Could you check a few things on this model? Use its own coordinates, in mm. A direction names the side the tool comes from. Coordinates: 2 decimals unless noted, no trailing zeros. Write each loop counter-clockwise with the first axis right and the second up, starting at its lowest first coordinate (ties: lowest second). Pieces come first, ordered by that corner, then holes.
```python
from build123d import *

# Parameters (mm, degrees)
SKETCH3_W          = 10
SKETCH3_H          = 1.5
CHAMFER1_SIZE      = 0.45
CUT_EXTRUDE1_DEPTH = 1.19


with BuildPart() as part:
    # Sketch3 → Revolve1 (revolve)
    with BuildSketch(Plane(origin=(0, 0, 0), x_dir=(0, 0, -1), z_dir=(1, 0, 0))):
        with Locations((0, 0.75)):
            Rectangle(SKETCH3_W, SKETCH3_H)
    revolve(axis=Axis((0, 0, -5), (0, 0, 1)))

    # Chamfer1
    chamfer1_edges = [part.edges().sort_by_distance(p)[0] for p in [
        (0, -1.5, -5),
    ]]
    chamfer(chamfer1_edges, length=CHAMFER1_SIZE)

    # Sketch6 → Revolve2 (revolve)
    with BuildSketch(Plane(origin=(0, 0, 0), x_dir=(0, 0, -1), z_dir=(1, 0, 0))):
        Polygon((-5, 3), (-4.8, 3), (-3.3, 1.5), (-3.3, 0), (-5, 0), align=None)
    revolve(axis=Axis((0, 0, -5), (0, 0, 1)))

    # Sketch8 → Cut-Extrude1 (cut)
    with BuildSketch(Plane.XY.offset(5)):
        Polygon((0, 1.154700538), (-1, 0.577350269), (-1, -0.577350269), (0, -1.154700538), (1, -0.577350269), (1, 0.577350269), align=None)
    extrude(amount=-CUT_EXTRUDE1_DEPTH, mode=Mode.SUBTRACT)

    # Cut-Extrude2 cone 1 section (through the dimple's axis) → Cut-Extrude2 (revolve, cut)
    with BuildSketch(Plane(origin=(0, 0, 5), x_dir=(0, -1, 0), z_dir=(1, 0, 0))):
        Polygon((0, 0), (1.154700538, 0), (0, 1.154700538), align=None)
    revolve(axis=Axis((0, 0, 5), (0, 0, -1)), mode=Mode.SUBTRACT)


solid = part.part
```
1. If we mould it in two halves opening along Y, with no side actions, what happens to faces 3 (the face through (0, 0, -5)), 4 (the face through (-0.07, -1.5, -0.68)), 5 (the face through (1, 0, 4))? For each: pulls with the +Y half, pulls with the -Y half, needs draft (parallel to the pull), parting line crosses it, or undercut.
Verdict:
face 3: needs draft
face 4: parting line crosses it
face 5: undercut
2. I want a section at A-A on y = 0. Please give me the cut outline in (x, z), plus the area to 3 significant figures.
Verdict:
outline: (-3, 4.8) - (-1.5, 3.3) - (-1.5, -4.55) - (-1.05, -5) - (1.05, -5) - (1.5, -4.55) - (1.5, 3.3) - (3, 4.8) - (3, 5) - (1.15, 5) - (1, 4.85) - (1, 3.81) - (-1, 3.81) - (-1, 4.85) - (-1.15, 5) - (-3, 5) - close
area: 30.2 mm2
3. On a 3-axis mill with a long thin cutter (end or side, diameter ignored), from which of +Z, -Z, +X, -X, +Y, -Y can I reach the whole of each face in a straight line? I mean faces 1 (the face through (0.51, 0.86, 4.41)), 2 (the face through (1, -1, 5)). Say none if no direction works.
Verdict:
face 1: +Z
face 2: +Z, +X, -X, +Y, -Y
4. I want a section at B-B on z = -3. Please give me the cut outline in (x, y), plus the area to 3 significant figures.
Verdict:
outline: circle Ø3 at (0, 0)
area: 7.07 mm2
5. Please list where these lines run through material, in increasing order: line 1 along Y through (x, z) = (0, -4.5); line 2 along Z through (x, y) = (-0.8, -2.3); line 3 along Z through (x, y) = (0, -1.8).
Verdict:
line 1: y = -1.5 to 1.5
line 2: z = 4.24 to 5
line 3: z = 3.6 to 5
6. For pin 1 (1.6 mm diameter, centred on x = 0, y = 0, fed in from +Z); pin 2 (3 mm diameter, centred on y = 2.5, z = -4, fed in from +X); pin 3 (1.5 mm diameter, centred on x = 0, z = -2, fed in from +Y), each with a flat end and sliding along its axis, tell me the tip position at first contact or that it passes through.
Verdict:
pin 1: stops at z = 3.81
pin 2: stops at x = 1.12
pin 3: stops at y = 1.5
